from build123d import *

# Parameters (mm, degrees)
SKETCH1_W           = 42.3
SKETCH1_H           = 42.3
BOSS_EXTRUDE1_DEPTH = 31
SKETCH2_R           = 1.644479294
CUT_EXTRUDE1_DEPTH  = 10
SKETCH3_R           = 11
BOSS_EXTRUDE2_DEPTH = 2
CHAMFER2_SIZE       = 5
SKETCH4_R           = 2
BOSS_EXTRUDE3_DEPTH = 150
SKETCH5_R           = 2.5
BOSS_EXTRUDE4_DEPTH = 13.5


with BuildPart() as part:
    # Sketch1 → Boss-Extrude1 (new body)
    with BuildSketch(Plane(origin=(0, 0, 0), x_dir=(1, 0, 0), z_dir=(0, 1, 0))):
        with Locations((21.15, 21.15)):
            Rectangle(SKETCH1_W, SKETCH1_H)
    extrude(amount=BOSS_EXTRUDE1_DEPTH)

    # Sketch2 → Cut-Extrude1 (cut)
    with BuildSketch(Plane(origin=(0, 31, 0), x_dir=(-1, 0, 0), z_dir=(0, 1, 0))):
        with Locations((-5.65, -36.65)):
            Circle(SKETCH2_R)
        with Locations((-36.65, -36.65)):
            Circle(SKETCH2_R)
        with Locations((-5.65, -5.65)):
            Circle(SKETCH2_R)
        with Locations((-36.65, -5.65)):
            Circle(SKETCH2_R)
    extrude(amount=-CUT_EXTRUDE1_DEPTH, mode=Mode.SUBTRACT)

    # Sketch3 → Boss-Extrude2 (add)
    with BuildSketch(Plane(origin=(0, 31, 0), x_dir=(-1, 0, 0), z_dir=(0, 1, 0))):
        with Locations((-21.15, -21.15)):
            Circle(SKETCH3_R)
    extrude(amount=BOSS_EXTRUDE2_DEPTH)

    # Chamfer2
    chamfer2_edges = [part.edges().sort_by_distance(p)[0] for p in [
        (0, 15.5, -42.3),
        (42.3, 15.5, -42.3),
        (42.3, 15.5, 0),
        (0, 15.5, 0),
    ]]
    chamfer(chamfer2_edges, length=CHAMFER2_SIZE)

    # Sketch4 → Boss-Extrude3 (add)
    with BuildSketch(Plane(origin=(0, 33, 0), x_dir=(-1, 0, 0), z_dir=(0, 1, 0))):
        with Locations((-21.15, -21.15)):
            Circle(SKETCH4_R)
    extrude(amount=BOSS_EXTRUDE3_DEPTH)

    # Sketch5 → Boss-Extrude4 (add)
    with BuildSketch(Plane.XZ):
        with Locations((21.15, -21.15)):
            Circle(SKETCH5_R)
    extrude(amount=BOSS_EXTRUDE4_DEPTH)


solid = part.part
CAD build for the part. Positions are in the model's coordinates, mm. A direction names the side the tool comes from. Give positions to 0.01 mm unless a question says otherwise; leave off trailing zeros. Write each loop counter-clockwise with the first axis right and the second up, starting at its lowest first coordinate (ties: lowest second). Pieces come first, ordered by that corner, then holes. Notation, with made-up numbers: M 37,10 L 69,10 A20 cw 69,43 Z; hole C -8,73.25 d9. An arc over 180 degrees is marked long. Put each result on its own line as item: value. Start each with the question number.
(1) Band-saw the part on A-A, the plane x = 21.15. Write the cut outline in (y, z), and give its area (3 significant figures).
(2) Flat gauge pins, fed straight in: pin 1 Ø4.5 at (x, z) = (36.65, -36.65) entering from -Y; pin 2 Ø3.5 at (x, z) = (6, -6) entering from +Y; pin 3 Ø2 at (x, z) = (36.65, -5.65) entering from +Y; pin 4 Ø10 at (x, y) = (30, 44) entering from -Z. Where does each tip first touch, or does it go through?
(3) Probe L1, parallel to Z at x = 36.65, y = 23.75; L2, parallel to Z at x = 4.5, y = 24; L3, parallel to Y at x = 11.5, z = -7. List the from-to ranges inside material, lowest first.
(4) Mould opens along Z. For faces 1 (the face through (6, 21, -37)), 2 (the face through (39.8, 15.3, -2.5)), 3 (the face through (32.14, 31.99, -20.67)) say: +Z half, -Z half, draft (parallel to the pull), parting line (faces both ways), or undercut.
(5) Band-saw the part on C-C, the plane z = -21.15. Write the cut outline in (x, y), and give its area (3 significant figures).
(6) Which spindle directions (+Z, -Z, +X, -X, +Y, -Y) get a long thin tool onto all of the face, cutting with end or side? Do faces 4 (the face through (42.3, 15, -21)), 5 (the face through (23.46, -6.66, -22.11)), 6 (the face through (30, 31, -12)). Say none if no direction does.
(7) Band-saw the part on D-D, the plane y = 158.5. Write the cut outline in (x, z), and give its area (3 significant figures).
(8) Band-saw the part on B-B, the plane y = 11. Write the cut outline in (x, z).
Response values:
1. outline: M -13.5,-23.65 L 0,-23.65 L 0,-42.3 L 31,-42.3 L 31,-32.15 L 33,-32.15 L 33,-23.15 L 183,-23.15 L 183,-19.15 L 33,-19.15 L 33,-10.15 L 31,-10.15 L 31,0 L 0,0 L 0,-18.65 L -13.5,-18.65 Z
1. area: 2,020 mm2
2. pin 1: stops at y = 0
2. pin 2: stops at y = 31
2. pin 3: stops at y = 21
2. pin 4: passes through
3. L1: z = -42.3 to -38.29, -35.01 to -7.29, -4.01 to 0
3. L2: z = -41.8 to -37.83, -35.47 to -6.83, -4.47 to -0.5
3. L3: y = 0 to 31
4. face 1: undercut
4. face 2: +Z half
4. face 3: parting line
5. outline: M 0,0 L 18.65,0 L 18.65,-13.5 L 23.65,-13.5 L 23.65,0 L 42.3,0 L 42.3,31 L 32.15,31 L 32.15,33 L 23.15,33 L 23.15,183 L 19.15,183 L 19.15,33 L 10.15,33 L 10.15,31 L 0,31 Z
5. area: 2,020 mm2
6. face 4: +Z, -Z, +X, +Y, -Y
6. face 5: -Y
6. face 6: +Y
7. outline: C 21.15,-21.15 d4
7. area: 12.6 mm2
8. outline: M 0,-37.3 L 5,-42.3 L 37.3,-42.3 L 42.3,-37.3 L 42.3,-5 L 37.3,0 L 5,0 L 0,-5 Z
